Check sheet for the drawn part. Datum: minimum x, y, z corner. Units: mm. A direction names the side the tool comes from. Coordinates: 2 decimals unless noted, no trailing zeros. Write each loop counter-clockwise with the first axis right and the second up, starting at its lowest first coordinate (ties: lowest second). Pieces come first, ordered by that corner, then holes. Notation, with made-up numbers: (36.5, 16.5) -> (52.5, 16.5) arc R7 cw to (52.5, 22.5) -> close; hole circle Ø7 at (-25, 60.5). An arc over 180 degrees is marked (long way). Write item = value, one per line. Start each with the question number.
(1) Section check D-D (z = 3.5). Record the cut outline in (x, y), plus the area to 3 significant figures.
(2) Mould release check, pull along X, two halves, no side actions. Record for the marked faces 3 and 4: released by +X, released by -X, zero draft, split by the parting line, or undercut.
(3) Gauge pin test, flat ends, axial feed: pin 1 Ø1 at (x, y) = (36, 0.5) entering from +Z; pin 2 Ø0.6 at (x, y) = (53.5, 1.5) entering from -Z; pin 3 Ø1.1 at (x, y) = (13, 3.5) entering from -Z. Record the tip position at first contact, or that the pin passes through.
(4) Section check A-A (y = 1.1). Record the cut outline in (x, z), plus the area to 3 significant figures.
(5) Section check C-C (z = 23). Record the cut outline in (x, y).
(6) Section check B-B (x = 53.5). Record the cut outline in (y, z).
(7) Set-up check for the marked faces 1 and 2: record each of +Z, -Z, +X, -X, +Y, -Y from which the full face is reachable in a straight line by a thin tool's end or side.
(8) Material ranges on probe 1 along X at (y, z) = (3.45, 18.5); probe 2 along X at (y, z) = (1.5, 16.5); probe 3 along Z at (x, y) = (9, 1.7), recorded low to high. Write a range as [from, to].
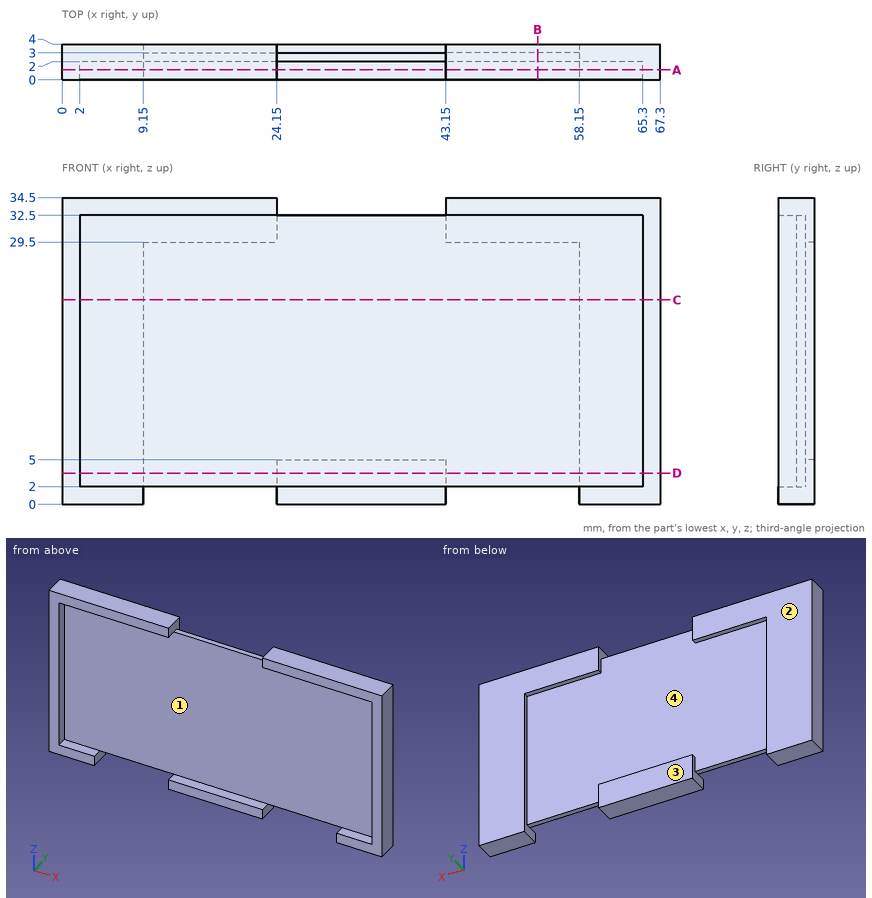
Response:
q1.outline = (0, 0) -> (2, 0) -> (2, 2) -> (65.3, 2) -> (65.3, 0) -> (67.3, 0) -> (67.3, 4) -> (58.15, 4) -> (58.15, 3) -> (43.15, 3) -> (43.15, 4) -> (24.15, 4) -> (24.15, 3) -> (9.15, 3) -> (9.15, 4) -> (0, 4) -> close
q1.area = 113 mm2
q2.face_3 = zero draft
q2.face_4 = undercut
q3.pin_1 = 2
q3.pin_2 = 32.5
q3.pin_3 = 2
q4.outline = (0, 0) -> (9.15, 0) -> (9.15, 2) -> (2, 2) -> (2, 32.5) -> (24.15, 32.5) -> (24.15, 34.5) -> (0, 34.5) -> close; (24.15, 0) -> (43.15, 0) -> (43.15, 2) -> (24.15, 2) -> close; (43.15, 32.5) -> (65.3, 32.5) -> (65.3, 2) -> (58.15, 2) -> (58.15, 0) -> (67.3, 0) -> (67.3, 34.5) -> (43.15, 34.5) -> close
q4.area = 293 mm2
q5.outline = (0, 0) -> (2, 0) -> (2, 2) -> (65.3, 2) -> (65.3, 0) -> (67.3, 0) -> (67.3, 4) -> (58.15, 4) -> (58.15, 3) -> (9.15, 3) -> (9.15, 4) -> (0, 4) -> close
q6.outline = (0, 32.5) -> (2, 32.5) -> (2, 2) -> (3, 2) -> (3, 29.5) -> (4, 29.5) -> (4, 34.5) -> (0, 34.5) -> close
q7.face_1 = -Y
q7.face_2 = +Z, -Z, +X, -X, +Y
q8.probe_1 = [0, 9.15], [58.15, 67.3]
q8.probe_2 = [0, 2], [65.3, 67.3]
q8.probe_3 = [0, 2], [32.5, 34.5]
